Here's the drawing with two shaded views (mm, measured from the low corner). I have some questions. A direction names the side the tool comes from. Coordinates: 2 decimals unless noted, no trailing zeros. Loops run counter-clockwise (first coordinate to the right, second up) from the corner with the lowest first, then second, coordinate; pieces in that order, holes last.
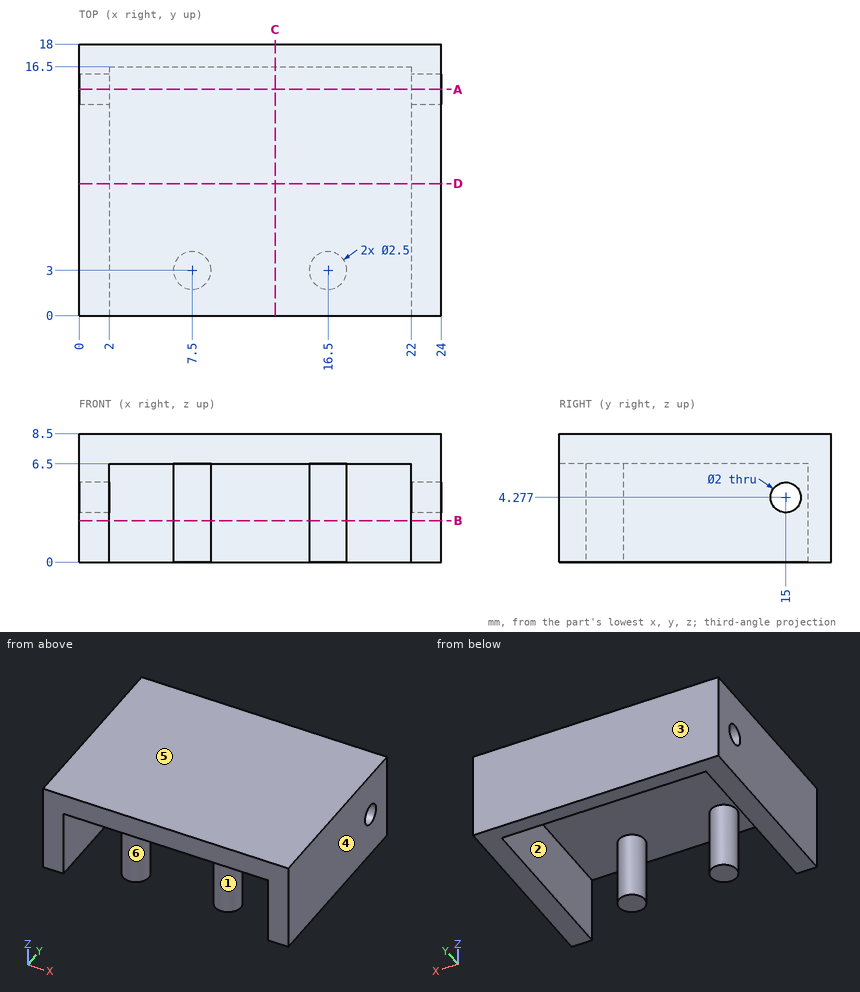
(1) I want a section at B-B on z = 2.75. Write out the boundary of the cut face in (x, y), then the cut area to 3 significant figures.
Check values:
outline: (0, 0) - (2, 0) - (2, 16.5) - (22, 16.5) - (22, 0) - (24, 0) - (24, 18) - (0, 18) - close; circle Ø2.5 at (7.5, 3); circle Ø2.5 at (16.5, 3)
area: 112 mm2
(2) If I drill on probe 1 along X at (y, z) = (14, 3.75); probe 2 along Z at (x, y) = (1.35, 15); probe 3 along Y at (x, z) = (2.25, 1), over which ranges is the centre line in solid material (lowest first)?
Check values:
probe 1: x = 0 to 2, 22 to 24
probe 2: z = 0 to 3.28, 5.28 to 8.5
probe 3: y = 16.5 to 18
(3) I want a section at C-C on x = 13. Write out the boundary of the cut face in (y, z).
Check values:
outline: (0, 6.5) - (16.5, 6.5) - (16.5, 0) - (18, 0) - (18, 8.5) - (0, 8.5) - close
(4) I want a section at A-A on y = 15. Write out the boundary of the cut face in (x, z).
Check values:
outline: (0, 0) - (2, 0) - (2, 3.28) - (0, 3.28) - close; (0, 5.28) - (2, 5.28) - (2, 6.5) - (22, 6.5) - (22, 5.28) - (24, 5.28) - (24, 8.5) - (0, 8.5) - close; (22, 0) - (24, 0) - (24, 3.28) - (22, 3.28) - close
(5) Which directions (+Z, -Z, +X, -X, +Y, -Y) give clear straight access to the entire face, cutting with the end or side of a thin tool? Please do the marked faces 1, 2 and 3.
Check values:
face 1: -Z
face 2: -Z, -Y
face 3: +Z, -Z, +X, -X, +Y
(6) I'm going to push flat-ended pins straight in: pin 1 (8 mm diameter, centred on x = 12, y = 11.5, fed in from -Z); pin 2 (2 mm diameter, centred on x = 7.5, z = 4, fed in from -Y); pin 3 (1.6 mm diameter, centred on y = 15, z = 4.28, fed in from +X); pin 4 (2 mm diameter, centred on x = 6.5, y = 3.5, fed in from -Z). Where does each tip first touch, or does it pass through?
Check values:
pin 1: stops at z = 6.5
pin 2: stops at y = 1.75
pin 3: passes through
pin 4: stops at z = 0
(7) I want a section at D-D on y = 8.75. Write out the boundary of the cut face in (x, z), then the cut area to 3 significant figures.
Check values:
outline: (0, 0) - (2, 0) - (2, 6.5) - (22, 6.5) - (22, 0) - (24, 0) - (24, 8.5) - (0, 8.5) - close
area: 74.0 mm2
(8) If we mould it in two halves opening along X, with no side actions, what happens to the marked faces 4, 5 and 6? For each: released by +X, released by -X, zero draft, split by the parting line, or undercut.
Check values:
face 4: released by +X
face 5: zero draft
face 6: undercut
